```python
from build123d import *

# Parameters (mm, degrees)
PAD_DEPTH       = 12
POCKET_DEPTH    = 1
FILLET_R        = 20
FILLET001_R     = 20
FILLET002_R     = 20
POCKET001_DEPTH = 5
SKETCH004_W     = 450
SKETCH004_H     = 12
PAD001_DEPTH    = 495
SKETCH005_W     = 300.149746
SKETCH005_H     = 18
PAD002_DEPTH    = 18


with BuildPart() as part:
    # Sketch001 → Pad (new body)
    with BuildSketch(Plane.XZ):
        Polygon((-20, -20), (-20, 110), (136.232082, 151.86226), (292.061476, 580), (480, 511.595971), (480, -20), align=None)
    extrude(amount=-PAD_DEPTH)

    # Sketch002 (on Face7 of Pad) → Pocket (cut)
    with BuildSketch(Plane.XZ):
        Polygon((465, -5), (465, 501.092858), (301.026563, 560.774309), (147.656805, 139.394363), (-5, 98.490095), (-5, -5), align=None)
    extrude(amount=POCKET_DEPTH, mode=Mode.SUBTRACT)

    # Fillet
    fillet_edges = [part.edges().sort_by_distance(p)[0] for p in [
        (-20, 6, 110),
    ]]
    fillet(fillet_edges, radius=FILLET_R)

    # Fillet001
    fillet001_edges = [part.edges().sort_by_distance(p)[0] for p in [
        (136.232082, 6, 151.86226),
    ]]
    fillet(fillet001_edges, radius=FILLET001_R)

    # Fillet002
    fillet002_edges = [part.edges().sort_by_distance(p)[0] for p in [
        (292.061476, 6, 580),
    ]]
    fillet(fillet002_edges, radius=FILLET002_R)

    # Sketch003 (on Face7 of Pocket) → Pocket001 (cut)
    with BuildSketch(Plane.XZ):
        Polygon((334.938299, 537.791251), (157.051626, 65.158909), (152.372098, 66.920163), (330.258771, 539.552506), align=None)
    extrude(amount=-POCKET001_DEPTH, mode=Mode.SUBTRACT)

    # Sketch004 (on Face11 of Pocket001) → Pad001 (join)
    with BuildSketch(Plane.XZ):
        with Locations((235, -4)):
            Rectangle(SKETCH004_W, SKETCH004_H)
    extrude(amount=PAD001_DEPTH)

    # Sketch005 (on Face1 of Pad001) → Pad002 (join)
    with BuildSketch(Plane.XZ):
        with Locations((309.925127, 11)):
            Rectangle(SKETCH005_W, SKETCH005_H)
    extrude(amount=PAD002_DEPTH)


solid = part.part
```
The listing builds one solid part. Answer for the finished solid, in the listing's coordinates (mm). A direction names the side the tool comes from. Give positions to 0.01 mm unless a question says otherwise; leave off trailing zeros. Loops run counter-clockwise (first coordinate to the right, second up) from the corner with the lowest first, then second, coordinate; pieces in that order, holes last. Notation, with made-up numbers: (-6.75, 19.25) - (44.25, 19.25) arc R13 cw to (44.25, 33.25) - close; hole circle Ø8 at (21.5, -15.5). An arc over 180 degrees is marked (long way). Answer as CSV lines item,"result". Start each with the question number.
Item 1: A cutting plane is placed at A-A on x = 372. Determine the outline of the cut face in (y, z).
Item 2: Find the intervals of material crossed by line 1 (Y direction, x = 284, z = 185.5); line 2 (Z direction, x = 327, y = -307), in increasing order. Write a range as from..to.
Item 3: A cutting plane is placed at D-D on x = 19. Determine the outline of the cut face in (y, z), then the cut area to 3 significant figures.
Item 4: The mould has two halves that part along X. Classify faces 5 (the face through (59.58, 5.916, 131.323)), 6 (the face through (308, -18, 11)), 7 (the face through (240.07, 2.46, 299.93)), 8 (the face through (394.24, 5.92, 542.81)): +X half, -X half, draft (parallel to the pull), parting line (faces both ways), or undercut.
Item 5: A cutting plane is placed at B-B on z = 225.5. Determine the outline of the cut face in (x, y), then the cut area to 3 significant figures.
Item 6: Each of these flat-tipped pins is pushed along its axis until it touches: pin 1 (12 mm diameter, centred on x = 350.5, y = -393, fed in from +Z); pin 2 (5 mm diameter, centred on x = 220, z = 354.5, fed in from -Y); pin 3 (13 mm diameter, centred on y = -332, z = -6, fed in from -X). Where does it stop, or does it pass through?
Item 7: A cutting plane is placed at C-C on y = -408. Determine the outline of the cut face in (x, z), then the cut area to 3 significant figures.
Item 8: For faces 1 (the face through (244, 5, 303)), 2 (the face through (308, -9, 20)), 3 (the face through (460, -244, -2)), 4 (the face through (159.85, -9, 11)), determine the directions among +Z, -Z, +X, -X, +Y, -Y from which every point of the face is accessible in a straight line to the end or side of a thin tool.
Found:
1,outline,"(-495, -10) - (0, -10) - (0, -20) - (12, -20) - (12, 550.9) - (0, 550.9) - (0, 20) - (-18, 20) - (-18, 2) - (-495, 2) - close"
2,line 1,"y = 0..12"
2,line 2,"z = -10..2"
3,outline,"(-495, -10) - (0, -10) - (0, -20) - (12, -20) - (12, 120.45) - (0, 120.45) - (0, 2) - (-495, 2) - close"
3,area,"7,630 mm^2"
4,face 5,"-X half"
4,face 6,"draft"
4,face 7,"undercut"
4,face 8,"+X half"
5,outline,"(163.03, 0) - (212.06, 0) - (212.06, 5) - (217.4, 5) - (217.4, 0) - (480, 0) - (480, 12) - (163.03, 12) - close"
5,area,"3,780 mm^2"
6,pin 1,"stops at z = 2"
6,pin 2,"stops at y = 0"
6,pin 3,"stops at x = 10"
7,outline,"(10, -10) - (460, -10) - (460, 2) - (10, 2) - close"
7,area,"5,400 mm^2"
8,face 1,"-Y"
8,face 2,"+Z, +X, -X, -Y"
8,face 3,"+Z, -Z, +X, -Y"
8,face 4,"+Z, -X, -Y"
